```python
from build123d import *

# Parameters (mm, degrees)
F0_W     = 7
F0_H     = 2
F1_DEPTH = 6
F2_R     = 1.75
F3_DEPTH = 5.001
F4_R     = 1.5


with BuildPart() as f1:
    # F0 (on Front) → F1 (new body)
    with BuildSketch(Plane.XZ):
        Polygon((5, 8), (5, 5), (12, 5), (21, 5), (28, 5), (28, 8), align=None)
        with Locations((8.5, 4)):
            Rectangle(F0_W, F0_H)
        with Locations((24.5, 4)):
            Rectangle(F0_W, F0_H)
    extrude(amount=F1_DEPTH)

    # F2 (on face) → F3 (cut, through all)
    with BuildSketch(Plane.XY.offset(8)):
        with Locations((9, -3)):
            Circle(F2_R)
        with Locations((24, -3)):
            Circle(F2_R)
    extrude(amount=-F3_DEPTH, mode=Mode.SUBTRACT)

    # F4
    f4_edges = [f1.edges().sort_by_distance(p)[0] for p in [
        (12, -3, 5),
        (21, -3, 5),
    ]]
    fillet(f4_edges, radius=F4_R)


solid = f1.part
```
Geometry: final body of the model. Coordinates: model frame, mm. A direction names the side the tool comes from. Round coordinates to 2 decimals unless told otherwise and drop trailing zeros. Order: outer loops, then holes, each group sorted by start corner. A loop starts at its lowest first (then second) coordinate and runs counter-clockwise, first axis right, second up. Notation, with made-up numbers: (42, 62) -> (46, 62) arc R25 cw to (46, 81) -> close; hole circle Ø8 at (-28, 56.25). An arc over 180 degrees is marked (long way). Use one line per item in the form item = value. Start each with the question number.
1. Cut plane B-B (z = 4.1). Return the cut outline in (x, y), then the cut area to 3 significant figures.
2. Pin query (flat end, axial travel): pin 1 Ø1.8 at (x, y) = (15.5, -2.5) entering from -Z; pin 2 Ø3 at (x, y) = (24, -3) entering from -Z. Return the tip coordinate at first contact, or that it passes through.
3. Reachability of faces 1 (the face through (12.43, -3.04, 4.55)), 2 (the face through (7, -3, 3)) from +Z, -Z, +X, -X, +Y, -Y: full face, straight path, thin tool, end or side. Return the list, or none.
4. Draft query along Y for faces 3 (the face through (16, 0, 6)), 4 (the face through (17, -3, 8)), 5 (the face through (22.25, -2.92, 5.54)), 6 (the face through (16, -6, 6)). Return one class per face: pulls with the +Y half, pulls with the -Y half, needs draft (parallel to the pull), parting line crosses it, or undercut.
5. Cut plane A-A (y = -3). Return the cut outline in (x, z).
6. Line query: probe 1 along Y at (x, z) = (9, 6.25); probe 2 along X at (y, z) = (-3.05, 6.3); probe 3 along X at (y, z) = (-2.4, 3.4). Output: solid intervals per line, ascending.
7. Cut plane D-D (y = -5.1). Return the cut outline in (x, z), then the cut area to 3 significant figures.
8. Cut plane C-C (x = 24). Return the cut outline in (y, z), then the cut area to 3 significant figures.
Solution:
q1.outline = (5, -6) -> (12.13, -6) -> (12.13, 0) -> (5, 0) -> close; (20.87, -6) -> (28, -6) -> (28, 0) -> (20.87, 0) -> close; hole circle Ø3.5 at (9, -3); hole circle Ø3.5 at (24, -3)
q1.area = 66.3 mm^2
q2.pin_1 = 5
q2.pin_2 = through
q3.face_1 = -Z, +Y, -Y
q3.face_2 = -Z, +X, -X, +Y, -Y
q4.face_3 = pulls with the +Y half
q4.face_4 = needs draft
q4.face_5 = undercut
q4.face_6 = pulls with the -Y half
q5.outline = (5, 3) -> (7.25, 3) -> (7.25, 8) -> (5, 8) -> close; (10.75, 3) -> (12, 3) -> (12, 3.5) arc R1.5 cw to (13.5, 5) -> (19.5, 5) arc R1.5 cw to (21, 3.5) -> (21, 3) -> (22.25, 3) -> (22.25, 8) -> (10.75, 8) -> close; (25.75, 3) -> (28, 3) -> (28, 8) -> (25.75, 8) -> close
q6.probe_1 = -6 to -4.75, -1.25 to 0
q6.probe_2 = 5 to 7.25, 10.75 to 22.25, 25.75 to 28
q6.probe_3 = 5 to 7.36, 10.64 to 12, 21 to 22.36, 25.64 to 28
q7.outline = (5, 3) -> (12, 3) -> (12, 3.5) arc R1.5 cw to (13.5, 5) -> (19.5, 5) arc R1.5 cw to (21, 3.5) -> (21, 3) -> (28, 3) -> (28, 8) -> (5, 8) -> close
q7.area = 98.0 mm^2
q8.outline = (-6, 3) -> (-4.75, 3) -> (-4.75, 8) -> (-6, 8) -> close; (-1.25, 3) -> (0, 3) -> (0, 8) -> (-1.25, 8) -> close
q8.area = 12.5 mm^2
